```python
from build123d import *

# Parameters (mm, degrees)
SKETCH1_R           = 7.5
SKETCH1_R_2         = 2.5
BOSS_EXTRUDE1_DEPTH = 5
SKETCH3_W           = 10
SKETCH3_H           = 15
BOSS_EXTRUDE2_DEPTH = 15
SKETCH4_R           = 2.5
CUT_EXTRUDE1_DEPTH  = 15
FILLET1_R           = 5


with BuildPart() as part:
    # Sketch1 → Boss-Extrude1 (new body)
    # profile 1 of 3: a face of its own
    with BuildSketch(Plane.XY):
        Circle(SKETCH1_R)
        Circle(SKETCH1_R_2, mode=Mode.SUBTRACT)
    # profile 2 of 3: a face of its own
    with BuildSketch(Plane.XY):
        with BuildLine():
            Line((75, 7.5), (0, 7.5))
            ThreePointArc((0, 7.5), (5.303300859, 5.303300859), (7.5, 0))
            ThreePointArc((7.5, 0), (5.303300859, -5.303300859), (0, -7.5))
            Line((0, -7.5), (75, -7.5))
            ThreePointArc((75, -7.5), (67.5, 0), (75, 7.5))
        make_face()
    # profile 3 of 3: a face of its own
    with BuildSketch(Plane.XY):
        with Locations((75, 0)):
            Circle(SKETCH1_R)
        with Locations((75, 0)):
            Circle(SKETCH1_R_2, mode=Mode.SUBTRACT)
    extrude(amount=BOSS_EXTRUDE1_DEPTH)

    # Sketch3 → Boss-Extrude2 (add)
    with BuildSketch(Plane(origin=(0, 7.5, 0), x_dir=(1, 0, 0), z_dir=(0, 1, 0))):
        with Locations((-2.5, 2.5)):
            Rectangle(SKETCH3_W, SKETCH3_H)
    extrude(amount=-BOSS_EXTRUDE2_DEPTH)

    # Sketch4 → Cut-Extrude1 (cut)
    with BuildSketch(Plane(origin=(0, 7.5, 0), x_dir=(1, 0, 0), z_dir=(0, 1, 0))):
        with Locations(Location((-2.5, 2.5, 0), (0, 0, 180))):
            Circle(SKETCH4_R)
    extrude(amount=-CUT_EXTRUDE1_DEPTH, mode=Mode.SUBTRACT)

    # Fillet1
    fillet1_edges = [part.edges().sort_by_distance(p)[0] for p in [
        (-7.5, -3.75, 5),
        (2.5, 0, 0),
        (2.5, 0, -10),
        (-7.5, 0, -10),
    ]]
    fillet(fillet1_edges, radius=FILLET1_R - 0.0001)  # a hair under: the kernel refuses the full size


solid = part.part
```
For this review, take the finished solid that the model builds, in its own axes (mm). A direction names the side the tool comes from. Round coordinates to 2 decimals unless told otherwise and drop trailing zeros. Write each loop counter-clockwise with the first axis right and the second up, starting at its lowest first coordinate (ties: lowest second). Pieces come first, ordered by that corner, then holes. Notation, with made-up numbers: M -31.75,61.5 L 11.25,61.5 A18 cw 11.25,85.5 Z; hole C -18,18.5 d5. An arc over 180 degrees is marked long. One line per item, written item: value. Start each with the question number.
(1) We need section A-A (y = 0). Count the separate pieces of the cut face and the enclosed holes in it, and give its area (3 significant figures).
(2) The part is to be moulded in two halves that separate along X. For faces 1 (the flat face through (33, -7.5, 1)), 2 (the cylindrical face through (1, -0.11, -8.57)), 3 (the cylindrical face through (-0.5, 0.1, -4)), say which applies: released by +X, released by -X, zero draft, split by the parting line, or undercut.
(3) Insertion check: pin 1 (3 mm diameter, centred on y = -6, z = -5.5, fed in from -X); pin 2 (6 mm diameter, centred on x = 49, y = 4, fed in from -Z). Each pin has a flat end and moves straight along its axis. Give the tip position at first contact, or say it passes through.
(4) Machinability: for faces 4 (the flat face through (33, 7.5, 1)), 5 (the flat face through (44, 0, 0)), which of the approach directions +Z, -Z, +X, -X, +Y, -Y give a long, thin tool a straight path to every point of the face, cutting with its end or side? Answer none if there is none.
(5) Wall thickness on line 1 (Z direction, x = -2.5, y = -0.5); line 2 (Y direction, x = 75, z = 2.95); line 3 (Z direction, x = 29, y = 2.5): over which ranges is each line inside the solid? List them lowest first.
(6) We need section D-D (z = 4.25). Give the boundary of the cut face in (x, y).
(7) We need section C-C (z = -0.75). Give the boundary of the cut face in (x, y).
Result:
1. separate pieces: 2
1. enclosed holes: 1
1. area: 495 mm²
2. face 1: zero draft
2. face 2: released by +X
2. face 3: undercut
3. pin 1: x = -7.5
3. pin 2: z = 0
4. face 4: +Z, -Z, +X, -X, +Y
4. face 5: -Z, +X, +Y, -Y
5. line 1: -10 to -5, 0 to 5
5. line 2: -7.5 to -2.5, 2.5 to 7.5
5. line 3: 0 to 5
6. outline: M -5.13,-7.5 L 75,-7.5 A7.5 ccw 75,7.5 L -5.13,7.5 Z; hole C 75,0 d5
7. outline: M -7.5,-7.5 L -4.29,-7.5 L -4.29,7.5 L -7.5,7.5 Z; M -0.71,-7.5 L 4.87,-7.5 L 4.87,7.5 L -0.71,7.5 Z
